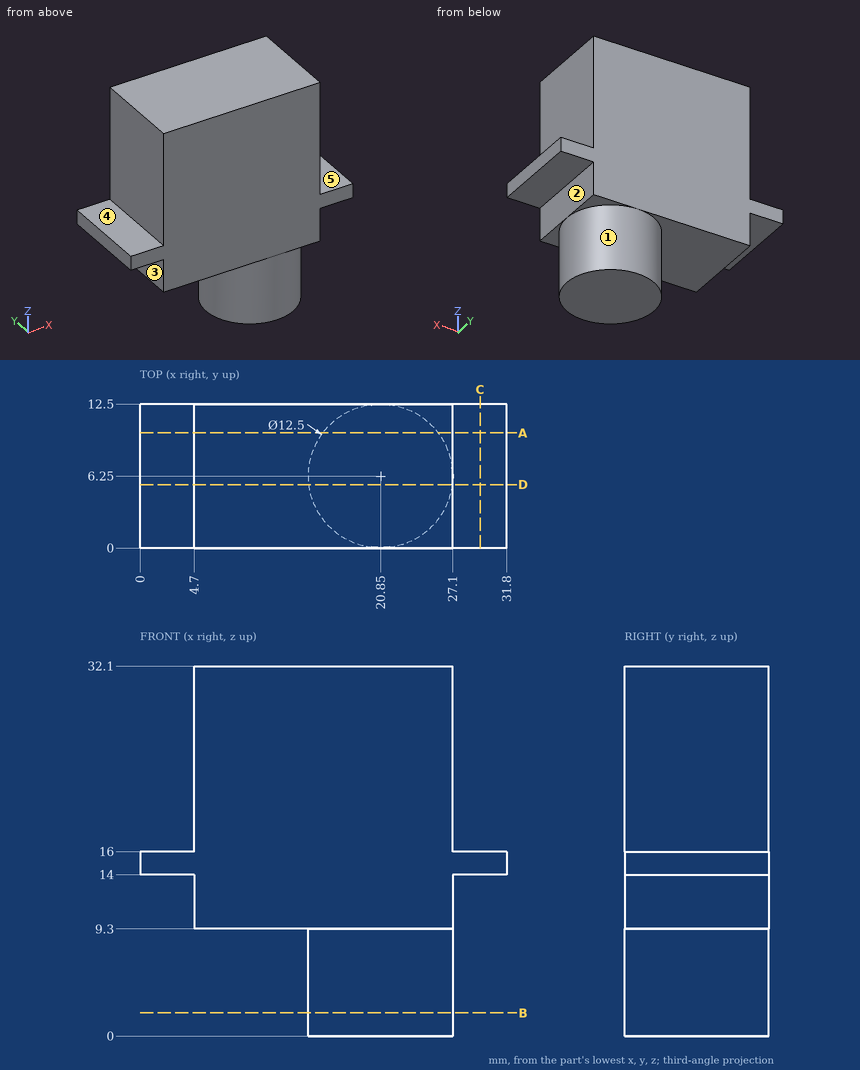
Input: dimensioned drawing with shaded views. Units: mm. Origin: part minimum x, y, z. A direction names the side the tool comes from. Round coordinates to 2 decimals unless told otherwise and drop trailing zeros. Order: outer loops, then holes, each group sorted by start corner. A loop starts at its lowest first (then second) coordinate and runs counter-clockwise, first axis right, second up.
1. Set-up query: the marked faces 1, 2, 3, 4 and 5. Return all of +Z, -Z, +X, -X, +Y, -Y with unobstructed straight access to the full face (end or side cutting, diameter ignored); none if empty.
The answers:
face 1: -Z
face 2: -Z, +X, +Y, -Y
face 3: -Z, -X, +Y, -Y
face 4: +Z, -X, +Y, -Y
face 5: +Z, +X, +Y, -Y
2. Cut plane D-D, the plane y = 5.5. Output: boundary loops of the cut face in (x, z).
The answers:
outline: (0, 14) - (4.7, 14) - (4.7, 9.3) - (14.65, 9.3) - (14.65, 0) - (27.05, 0) - (27.05, 9.3) - (27.1, 9.3) - (27.1, 14) - (31.8, 14) - (31.8, 16) - (27.1, 16) - (27.1, 32.1) - (4.7, 32.1) - (4.7, 16) - (0, 16) - close
3. Cut plane B-B, the plane z = 2. Output: boundary loops of the cut face in (x, y).
The answers:
outline: circle Ø12.5 at (20.85, 6.25)
4. Material intervals for line 1 (X direction, y = 8.5, z = 24); line 2 (Z direction, x = 12.5, y = 4.75); line 3 (Z direction, x = 3, y = 10), sorted ascending.
The answers:
line 1: x = 4.7 to 27.1
line 2: z = 9.3 to 32.1
line 3: z = 14 to 16
5. Pin query (flat end, axial travel): P1, Ø2.5, axis at y = 5, z = 11.5, coming from the +X side; P2, Ø4, axis at x = 30, y = 9, coming from the +Z side; P3, Ø5, axis at y = 6.5, z = 10.5, coming from the -X side. Return the tip coordinate at first contact, or that it passes through.
The answers:
P1: stops at x = 27.1
P2: stops at z = 16
P3: stops at x = 4.7
6. Cut plane A-A, the plane y = 10. Output: boundary loops of the cut face in (x, z), then the cut area to 3 significant figures.
The answers:
outline: (0, 14) - (4.7, 14) - (4.7, 9.3) - (15.85, 9.3) - (15.85, 0) - (25.85, 0) - (25.85, 9.3) - (27.1, 9.3) - (27.1, 14) - (31.8, 14) - (31.8, 16) - (27.1, 16) - (27.1, 32.1) - (4.7, 32.1) - (4.7, 16) - (0, 16) - close
area: 623 mm2
7. Cut plane C-C, the plane x = 29.5. Output: boundary loops of the cut face in (y, z).
The answers:
outline: (0, 14) - (12.5, 14) - (12.5, 16) - (0, 16) - close
